```python
from build123d import *

# Parameters (mm, degrees)
SKETCH1_W                       = 49.784
SKETCH1_H                       = 35.56
BOSS_EXTRUDE1_DEPTH             = 50.8
M4X0_7_TAPPED_HOLE1_AT_2_COUNT  = 2
M4X0_7_TAPPED_HOLE1_AT_2_PITCH  = 30
M4X0_7_TAPPED_HOLE1_AT_3_COUNT  = 2
M4X0_7_TAPPED_HOLE1_AT_3_PITCH  = 18
M4X0_7_TAPPED_HOLE1_AT_4_COUNT  = 2
M4X0_7_TAPPED_HOLE1_AT_4_PITCH  = 24
CUT_EXTRUDE2_DEPTH              = 0.508
MIRROR2_START                   = -17.78
MIRROR2_DEPTH                   = 0.508
M5X0_8_TAPPED_HOLE1_D           = 4.2
M5X0_8_TAPPED_HOLE1_DEPTH       = 12.192
M5X0_8_TAPPED_HOLE1_CSINK_D     = 6
M5X0_8_TAPPED_HOLE1_CSINK_ANGLE = 90
M5X0_8_TAPPED_HOLE1_TIP         = 1.2618073


# Read off the part's stored shape, not the designer's step: Mirror2
with BuildPart() as part:
    # Sketch1 → Boss-Extrude1 (new body)
    with BuildSketch(Plane.YZ):
        Rectangle(SKETCH1_W, SKETCH1_H)
    extrude(amount=BOSS_EXTRUDE1_DEPTH)

    # Sketch3 → M4x0.7 Tapped Hole1 (revolve, cut)
    with BuildSketch(Plane(origin=(13.4, -24.892, -9), x_dir=(0, 0, -1), z_dir=(1, 0, 0))):
        Polygon((0, 0), (0, 10.897420021), (1.65, 9.906), (1.65, 0.85), (2.5, 0), align=None)
    m4x0_7_tapped_hole1 = revolve(axis=Axis((13.4, -31.242, -9), (0, 1, 0)), mode=Mode.SUBTRACT)

    # M4x0.7 Tapped Hole1 at 2: M4x0.7 Tapped Hole1 ×2
    with Locations(*[Vector(0.8000000000000002, 0, 0.5999999999999998) * (i * M4X0_7_TAPPED_HOLE1_AT_2_PITCH) for i in range(1, M4X0_7_TAPPED_HOLE1_AT_2_COUNT)]):
        add(m4x0_7_tapped_hole1, mode=Mode.SUBTRACT)

    # M4x0.7 Tapped Hole1 at 3: M4x0.7 Tapped Hole1 ×2
    with Locations(*[(0, 0, i * M4X0_7_TAPPED_HOLE1_AT_3_PITCH) for i in range(1, M4X0_7_TAPPED_HOLE1_AT_3_COUNT)]):
        add(m4x0_7_tapped_hole1, mode=Mode.SUBTRACT)

    # M4x0.7 Tapped Hole1 at 4: M4x0.7 Tapped Hole1 ×2
    with Locations(*[(i * M4X0_7_TAPPED_HOLE1_AT_4_PITCH, 0, 0) for i in range(1, M4X0_7_TAPPED_HOLE1_AT_4_COUNT)]):
        add(m4x0_7_tapped_hole1, mode=Mode.SUBTRACT)

    # Mirror1: M4x0.7 Tapped Hole1 across plane
    add(m4x0_7_tapped_hole1.mirror(Plane.ZX), mode=Mode.SUBTRACT)

    # Mirror1 copy 1 sketch → Mirror1 copy 1 (revolve, cut)
    with BuildSketch(Plane(origin=(37.4, 24.892, 9), x_dir=(0, 0, -1), z_dir=(1, 0, 0))):
        Polygon((0, 0), (0, -10.897420021), (1.65, -9.906), (1.65, -0.85), (2.5, 0), align=None)
    revolve(axis=Axis((37.4, 31.242, 9), (0, 1, 0)), mode=Mode.SUBTRACT)

    # Mirror1 copy 2 sketch → Mirror1 copy 2 (revolve, cut)
    with BuildSketch(Plane(origin=(13.4, 24.892, 9), x_dir=(0, 0, -1), z_dir=(1, 0, 0))):
        Polygon((0, 0), (0, -10.897420021), (1.65, -9.906), (1.65, -0.85), (2.5, 0), align=None)
    revolve(axis=Axis((13.4, 31.242, 9), (0, 1, 0)), mode=Mode.SUBTRACT)

    # Mirror1 copy 3 sketch → Mirror1 copy 3 (revolve, cut)
    with BuildSketch(Plane(origin=(37.4, 24.892, -9), x_dir=(0, 0, -1), z_dir=(1, 0, 0))):
        Polygon((0, 0), (0, -10.897420021), (1.65, -9.906), (1.65, -0.85), (2.5, 0), align=None)
    revolve(axis=Axis((37.4, 31.242, -9), (0, 1, 0)), mode=Mode.SUBTRACT)

    # Sketch5 → Cut-Revolve1 (revolve, cut)
    with BuildSketch(Plane(origin=(0, 0, 0), x_dir=(-1, 0, 0), z_dir=(0, 1, 0))):
        Polygon((-25.4, 17.78), (-25.4, 13.964535069), (-31.75, 17.78), align=None)
    revolve(axis=Axis((25.4, 0, 17.78), (0, 0, -1)), mode=Mode.SUBTRACT)

    # Sketch9 → Cut-Extrude2 (cut)
    with BuildSketch(Plane(origin=(0, 0, -17.78), x_dir=(1, 0, 0), z_dir=(0, 0, -1))):
        with BuildLine():
            Line((25.4, 12.7), (31.75, 12.7))
            ThreePointArc((31.75, 12.7), (34.925, 15.875), (38.1, 12.7))
            Line((38.1, 12.7), (38.1, 9.652))
            Line((38.1, 9.652), (50.8, 9.652))
            Line((50.8, 9.652), (50.8, 0))
            Line((50.8, 0), (25.4, 0))
            Line((25.4, 0), (25.4, 12.7))
        make_face()
    extrude(amount=-CUT_EXTRUDE2_DEPTH, mode=Mode.SUBTRACT)

    # Mirror2 outline → Mirror2 (cut)
    with BuildSketch(Plane.XY.offset(MIRROR2_START)):
        with BuildLine():
            Line((38.1, 9.652), (38.1, 12.7))
            ThreePointArc((38.1, 12.7), (34.925, 15.875), (31.75, 12.7))
            Line((31.75, 12.7), (19.05, 12.7))
            ThreePointArc((19.05, 12.7), (15.875, 15.875), (12.7, 12.7))
            Line((12.7, 12.7), (12.7, 9.652))
            Line((12.7, 9.652), (0, 9.652))
            Line((0, 9.652), (0, -9.652))
            Line((0, -9.652), (12.7, -9.652))
            Line((12.7, -9.652), (12.7, -12.7))
            ThreePointArc((12.7, -12.7), (15.875, -15.875), (19.05, -12.7))
            Line((19.05, -12.7), (25.4, -12.7))
            Line((25.4, -12.7), (25.4, 0))
            Line((25.4, 0), (50.8, 0))
            Line((50.8, 0), (50.8, 9.652))
            Line((50.8, 9.652), (38.1, 9.652))
        make_face()
    extrude(amount=MIRROR2_DEPTH, mode=Mode.SUBTRACT)

    # M5x0.8 Tapped Hole1
    with Locations(Plane(origin=(0, 0, -17.272), x_dir=(1, 0, 0), z_dir=(0, 0, -1))):
        with Locations((44.45, 0)):
            CounterSinkHole(M5X0_8_TAPPED_HOLE1_D / 2, M5X0_8_TAPPED_HOLE1_CSINK_D / 2, depth=M5X0_8_TAPPED_HOLE1_DEPTH, counter_sink_angle=M5X0_8_TAPPED_HOLE1_CSINK_ANGLE)
            with Locations((0, 0, -(M5X0_8_TAPPED_HOLE1_DEPTH + M5X0_8_TAPPED_HOLE1_TIP / 2))):  # 118° drill point
                Cone(0, M5X0_8_TAPPED_HOLE1_D / 2, M5X0_8_TAPPED_HOLE1_TIP, mode=Mode.SUBTRACT)


solid = part.part
```
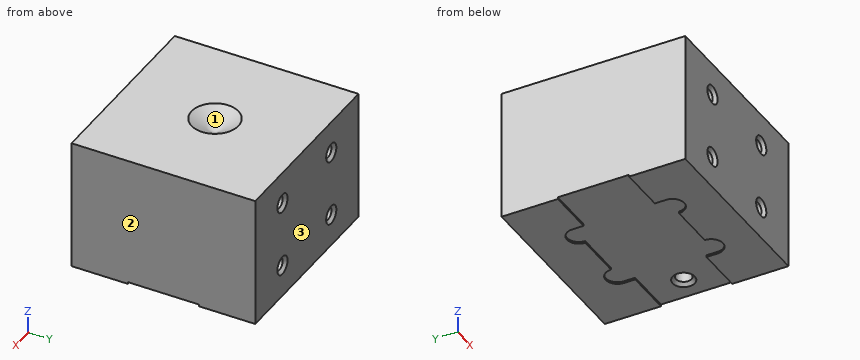
Verification items for the finished model (mm, model axes). Face numbers are marked on the shaded views. Round coordinates to 2 decimals unless told otherwise and drop trailing zeros. Order: outer loops, then holes, each group sorted by start corner. A loop starts at its lowest first (then second) coordinate and runs counter-clockwise, first axis right, second up.
1) Cross-section at A-A, the plane y = 20.5. Record the cut outline in (x, z).
Geometry says:
outline: (0, -17.78) - (50.8, -17.78) - (50.8, 17.78) - (0, 17.78) - close; hole circle Ø3.3 at (13.4, -9); hole circle Ø3.3 at (13.4, 9); hole circle Ø3.3 at (37.4, -9); hole circle Ø3.3 at (37.4, 9)
2) Depth check by flat-ended pin: pin 1 (6 mm diameter, centred on y = -4.5, z = -14, fed in from -X); pin 2 (3 mm diameter, centred on x = 37.4, z = 9, fed in from -Y); pin 3 (2 mm diameter, centred on x = 13.4, z = -9, fed in from -Y); pin 4 (2 mm diameter, centred on x = 37.4, z = -9, fed in from +Y). Enter the tip coordinate at first touch or a pass-through.
Geometry says:
pin 1: stops at x = 0
pin 2: stops at y = -14.9
pin 3: stops at y = -14.6
pin 4: stops at y = 14.6
3) Material ranges on line 1 (X direction, y = -20.25, z = -9); line 2 (Y direction, x = 44.45, z = -11.25); line 3 (Z direction, x = 38, y = 21.5), recorded low to high.
Geometry says:
line 1: x = 0 to 11.75, 15.05 to 35.75, 39.05 to 50.8
line 2: y = -24.89 to -2.1, 2.1 to 24.89
line 3: z = -17.78 to -10.54, -7.46 to 7.46, 10.54 to 17.78
4) Draft check along Y on the marked faces 1, 2 and 3. Enter one of: +Y half, -Y half, draft (parallel to the pull), parting line (faces both ways), or undercut.
Geometry says:
face 1: undercut
face 2: draft
face 3: +Y half
